Autodesk Inventor part; units mm, degrees
ref_plane "YZ Plane" through (0, 0, 0) normal (1, 0, 0) x (0, 1, 0)
ref_plane "XZ Plane" through (0, 0, 0) normal (0, 1, 0) x (-1, 0, 0)
ref_plane "XY Plane" through (0, 0, 0) normal (0, 0, 1) x (1, 0, 0)
sketch "Sketch1" plane through (0, 0, 0) normal (0, 0, 1) x (1, 0, 0)
  circle A0 centre (0, 0) radius 15
  circle A1 centre (0, 0) radius 25
  dimension "d0" = 30
extrude "Extrusion1" add sketch "Sketch1" along normal mid plane 30
extrude "Extrusion2" add sketch "Sketch1" against normal blind 10 contours A0
extrude "Extrusion3" add sketch "Sketch1" along normal blind 40 contours A0
chamfer "Chamfer1" distance 2 angle 45 1 edges at (-25, 0, 15)
sketch "Sketch2" plane through (0, 0, -15) normal (0, 0, -1) x (-1, 0, 0)
  circle A0 centre (0, 0) radius 25
  circle A1 centre (0, 0) radius 15
  line L0 (-22.5, 3) -> (-25.5, 3)
  line L1 (-25.5, 3) -> (-25.5, -3)
  line L2 (-25.5, -3) -> (-22.5, -3)
  line L3 (-22.5, -3) -> (-22.5, 3)
  line L4 (-22.5, 3) -> (-25.5, -3) construction
  line L5 (-25.5, 3) -> (-22.5, -3) construction
  point P0 (-24, 0)
  dimension "d12" = 6
  dimension "d13" = 24
  dimension "d14" = 3
extrude "Extrusion4" cut sketch "Sketch2" against normal through all contours L0 L3 L2 A0 | A0 L2 L1 L0 picked at (-23.3266, 0.334)
chamfer "Chamfer2" distance 2 angle 45 5 edges at (24.8193, -3, -1) (24.8193, 3, -1) (22.5, 0, -15) (22.5, 0, 15) (-15, 0, 40)
pattern_circular "Circular Pattern1" count 6 over 360 about axis through (0, 0, -10) along (0, 0, 1) of "Extrusion4"
sketch "Sketch3" plane through (0, 0, 15) normal (0, 0, 1) x (1, 0, 0)
  circle A0 centre (0, 0) radius 15
  line L0 (20.5, 3) -> (20.5, -3)
  line L1 (20.5, -3) -> (22.8035, -3)
  arc A1 (13.9998, -18.2484) -> (22.8035, -3) centre (0, 0) ccw
  line L2 (13.9998, -18.2484) -> (13.8481, -17.9856)
  line L3 (13.8481, -17.9856) -> (8.6519, -20.9856)
  line L4 (8.6519, -20.9856) -> (8.8037, -21.2484)
  arc A2 (-8.8037, -21.2484) -> (8.8037, -21.2484) centre (0, 0) ccw
  line L5 (-8.8037, -21.2484) -> (-8.6519, -20.9856)
  line L6 (-8.6519, -20.9856) -> (-13.8481, -17.9856)
  line L7 (-13.8481, -17.9856) -> (-13.9998, -18.2484)
  arc A3 (-22.8035, -3) -> (-13.9998, -18.2484) centre (0, 0) ccw
  line L8 (-22.8035, -3) -> (-22.5, -3)
  line L9 (-22.5, -3) -> (-22.5, 3)
  line L10 (-22.5, 3) -> (-22.8035, 3)
  arc A4 (-13.9998, 18.2484) -> (-22.8035, 3) centre (0, 0) ccw
  line L11 (-13.9998, 18.2484) -> (-13.8481, 17.9856)
  line L12 (-13.8481, 17.9856) -> (-8.6519, 20.9856)
  line L13 (-8.6519, 20.9856) -> (-8.8037, 21.2484)
  arc A5 (8.8037, 21.2484) -> (-8.8037, 21.2484) centre (0, 0) ccw
  line L14 (8.8037, 21.2484) -> (8.6519, 20.9856)
  line L15 (8.6519, 20.9856) -> (13.8481, 17.9856)
  line L16 (13.8481, 17.9856) -> (13.9998, 18.2484)
  arc A6 (22.8035, 3) -> (13.9998, 18.2484) centre (0, 0) ccw
  line L17 (22.8035, 3) -> (20.5, 3)
  circle A7 centre (0, 0) radius 17.5
  dimension "d21" = 35
extrude "Extrusion5" add sketch "Sketch3" along normal blind 5 contours A7
sketch "Sketch4" plane through (0, 0, 0) normal (1, 0, 0) x (0, 1, 0)
  line L0 (15, 20) -> (-15, 20)
  line L1 (15, 38) -> (-15, 38)
  line L2 (17.5, 20) -> (-17.5, 20)
  line L3 (-17.5, 15) -> (17.5, 15)
  line L4 (-19.9942, 13) -> (-19.9942, -15)
  line L5 (-4.9744, -15) -> (-19.9942, -15)
  line L6 (-4.9744, 13) -> (-4.9744, -15)
  line L7 (-19.9942, 13) -> (-4.9744, 13)
  line L8 (-15, 20) -> (-17.5, 15)
  line L9 (-18.2484, 15) -> (-3, 15)
  line L10 (-15, 15) -> (-15, 20)
  line L11 (-17.5, 15) -> (-15, 15)
  line L12 (-15, 20) -> (-17.5, 20)
  line L13 (-17.5, 20) -> (-17.5, 15)
  line L14 (-17.5, 15) -> (-15, 15)
  line L15 (-15, 15) -> (-15, 20)
  line L16 (0, -26) -> (0, 51)
  point P0 (0, 0)
revolve "Revolution1" cut sketch "Sketch4" angle 360 about axis through (0, 0, -10) along (0, 0, 1) contours L8 L13 L2
properties part number "base_hydraulic_pump" material "Stainless Steel"
Part model, mm, in its own coordinate system. A direction names the side the tool comes from. Round coordinates to 2 decimals unless told otherwise and drop trailing zeros. Loops run counter-clockwise (first coordinate to the right, second up) from the corner with the lowest first, then second, coordinate; pieces in that order, holes last.
Item 1: Cut at A-A, the plane x = 0. Give the cut face in (y, z), then the cut area to 3 significant figures.
Item 2: Cut at C-C, the plane z = -1.5. Give the cut face in (x, y).
Item 3: Cut at D-D, the plane z = 25.5. Give the cut face in (x, y), then the cut area to 3 significant figures.
Item 4: Cut at B-B, the plane y = 0. Give the cut face in (x, z), then the cut area to 3 significant figures.
Item 5: Drill centre lines: line 1 (Z direction, x = 0, y = -2); line 2 (Z direction, x = 12.5, y = 17.5); line 3 (X direction, y = 0.5, z = 7). Where is each one in solid material? Low to high.
Item 6: 3-axis set-ups, long thin cutter, end or side, ignore diameter. For faces 1 (the face through (21.5, 0, -14)), 2 (the face through (-14.985, 0.66, -12.465)), 3 (the face through (14.42, -18.98, -0.21)), 4 (the face through (11.21, -19.51, -0.21)), 5 (the face through (22.5, 0, 0)): which of +Z, -Z, +X, -X, +Y, -Y reach the whole face in a straight line?
Item 7: Mould opens along Y. For faces 6 (the face through (20.47, 12.12, 14.21)), 7 (the face through (-11, -11, -15)), 8 (the face through (-24, 3, 0)) say: +Y half, -Y half, draft (parallel to the pull), parting line (faces both ways), or undercut.
Item 8: Drop flat-ended pins along their axis: P1, Ø1.2, axis at x = 21.5, z = 3, coming from the -Y side; P2, Ø1, axis at x = 4, y = -9.5, coming from the -Z side; P3, Ø6.5, axis at y = 0, z = -5, coming from the -X side. Give the stop position or say it passes through.
A:
1. outline: (-25, -15) - (-15, -15) - (-15, -10) - (15, -10) - (15, -15) - (25, -15) - (25, 13) - (23, 15) - (17.5, 15) - (15, 20) - (15, 38) - (13, 40) - (-13, 40) - (-15, 38) - (-15, 20) - (-17.5, 15) - (-23, 15) - (-25, 13) - close
1. area: 2,100 mm2
2. outline: (-24.82, -3) arc R25 ccw to (-15.01, -19.99) - (-13.85, -17.99) - (-8.65, -20.99) - (-9.81, -22.99) arc R25 ccw to (9.81, -22.99) - (8.65, -20.99) - (13.85, -17.99) - (15.01, -19.99) arc R25 ccw to (24.5, -4.97) - (22.82, -3) - (22.5, -3) - (22.5, 3) - (22.82, 3) - (24.5, 4.97) arc R25 ccw to (15.01, 19.99) - (13.85, 17.99) - (8.65, 20.99) - (9.81, 22.99) arc R25 ccw to (-9.81, 22.99) - (-8.65, 20.99) - (-13.85, 17.99) - (-15.01, 19.99) arc R25 ccw to (-24.82, 3) - (-22.5, 3) - (-22.5, -3) - close
3. outline: circle Ø30 at (0, 0)
3. area: 707 mm2
4. outline: (-22.5, -15) - (-15, -15) - (-15, -10) - (15, -10) - (15, -15) - (20.5, -15) - (22.5, -13) - (22.5, 13) - (20.5, 15) - (17.5, 15) - (15, 20) - (15, 38) - (13, 40) - (-13, 40) - (-15, 38) - (-15, 20) - (-17.5, 15) - (-22.5, 15) - close
4. area: 1,950 mm2
5. line 1: z = -10 to 40
5. line 2: z = -15 to 15
5. line 3: x = -22.5 to 22.5
6. face 1: -Z, +X
6. face 2: -Z
6. face 3: +Z, -Z, -Y
6. face 4: +Z, -Z
6. face 5: +Z, -Z, +X
7. face 6: +Y half
7. face 7: draft
7. face 8: undercut
8. P1: stops at y = -13.72
8. P2: stops at z = -10
8. P3: stops at x = -24.82
